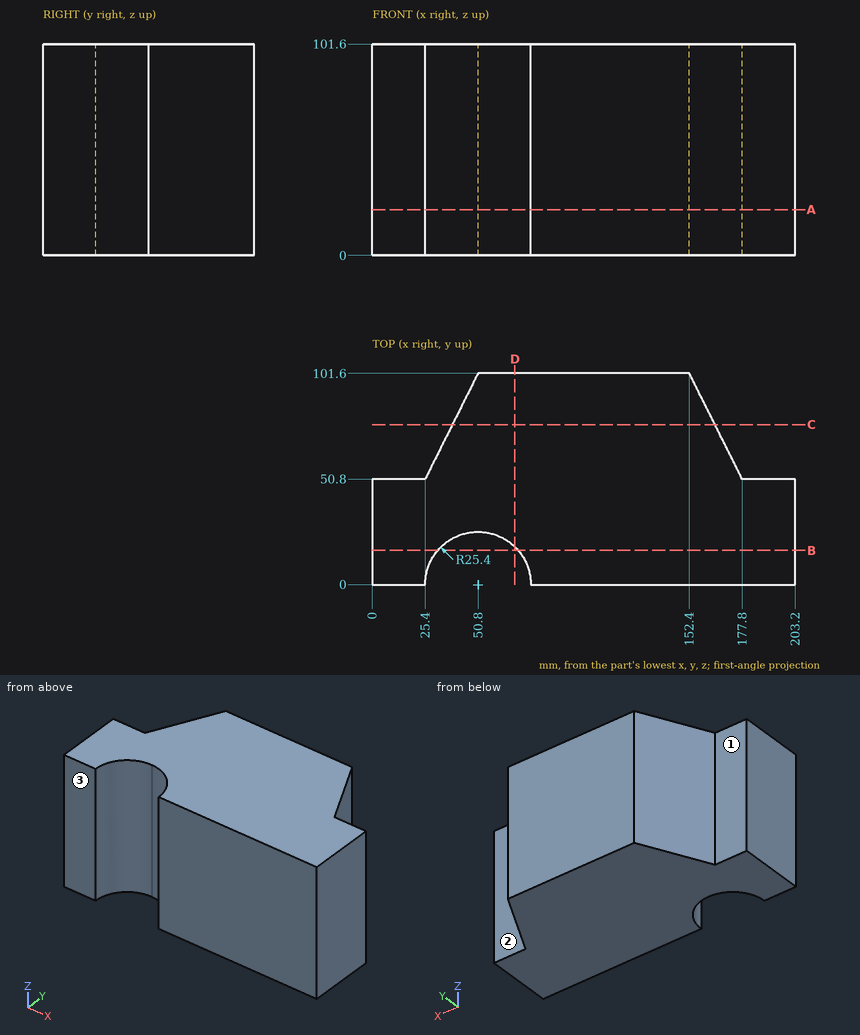
Print and shaded views of the part. All mm, measured from the part's lowest x, y and z. A direction names the side the tool comes from. Coordinates: 2 decimals unless noted, no trailing zeros. Order: outer loops, then holes, each group sorted by start corner. A loop starts at its lowest first (then second) coordinate and runs counter-clockwise, first axis right, second up. Notation, with made-up numbers: (-12, -2.5) - (46, -2.5) arc R11 ccw to (46, 16.5) - close; hole circle Ø5 at (67, 52). An arc over 180 degrees is marked (long way). Put each result on its own line as item: value.
1. Saw through at D-D (x = 68.5). Write the cut outline in (y, z), and give its area (3 significant figures).
Answer sheet:
outline: (18.22, 0) - (101.6, 0) - (101.6, 101.6) - (18.22, 101.6) - close
area: 8,470 mm^2
2. Saw through at A-A (z = 22). Write the cut outline in (x, y).
Answer sheet:
outline: (0, 0) - (25.4, 0) arc R25.4 cw to (76.2, 0) - (203.2, 0) - (203.2, 50.8) - (177.8, 50.8) - (152.4, 101.6) - (50.8, 101.6) - (25.4, 50.8) - (0, 50.8) - close
3. Tool access for the marked faces 1, 2 and 3: list every direction of +Z, -Z, +X, -X, +Y, -Y with a clear straight run to the whole face (end or side of a thin tool).
Answer sheet:
face 1: +Z, -Z, -X, +Y
face 2: +Z, -Z, +X, +Y
face 3: +Z, -Z, +X, -X, -Y
4. Drop flat-ended pins along their axis: P1, Ø6, axis at x = 141, y = 27, coming from the -Z side; P2, Ø10, axis at x = 54.5, z = 31.5, coming from the -Y side. Give the stop position or say it passes through.
Answer sheet:
P1: stops at z = 0
P2: stops at y = 23.86
5. Probe line 1 along X through (y, z) = (79, 43.5); line 2 along X through (y, z) = (58, 82.5); line 3 along X through (y, z) = (18.5, 53.5). List the from-to ranges inside material, lowest first. Write a range as [from, to].
Answer sheet:
line 1: x = [39.5, 163.7]
line 2: x = [29, 174.2]
line 3: x = [0, 33.4], [68.2, 203.2]
6. Saw through at B-B (y = 16.5). Write the cut outline in (x, z), and give its area (3 significant figures).
Answer sheet:
outline: (0, 0) - (31.49, 0) - (31.49, 101.6) - (0, 101.6) - close; (70.11, 0) - (203.2, 0) - (203.2, 101.6) - (70.11, 101.6) - close
area: 16,700 mm^2
7. Saw through at C-C (y = 77). Write the cut outline in (x, z), and give its area (3 significant figures).
Answer sheet:
outline: (38.5, 0) - (164.7, 0) - (164.7, 101.6) - (38.5, 101.6) - close
area: 12,800 mm^2
